Design review of the part built by this model. Coordinates are the model's own, in mm. A direction names the side the tool comes from. Coordinates: 2 decimals unless noted, no trailing zeros. Loops run counter-clockwise (first coordinate to the right, second up) from the corner with the lowest first, then second, coordinate; pieces in that order, holes last. Notation, with made-up numbers: (-25, -29.5) -> (5, -29.5) arc R21 ccw to (5, -22.5) -> close; hole circle Ø4 at (-33.75, 66.5). An arc over 180 degrees is marked (long way). Answer in a Markdown table with one row per item.
```python
from build123d import *

# Parameters (mm, degrees)
BOSS_EXTRUDE1_DEPTH = 12.7
SKETCH2_R           = 3.175
CUT_EXTRUDE1_DEPTH  = 12.7


with BuildPart() as part:
    # Sketch1 → Boss-Extrude1 (new body)
    with BuildSketch(Plane.XY):
        with BuildLine():
            Line((-25.4, 6.391326247), (-25.4, 34.062325918))
            ThreePointArc((-25.4, 34.062325918), (-50.8, 59.462325918), (-76.2, 34.062325918))
            Line((-76.2, 34.062325918), (-101.6, 34.062325918))
            ThreePointArc((-101.6, 34.062325918), (-50.8, 84.862325918), (0, 34.062325918))
            Line((0, 34.062325918), (0, 0))
            Line((0, 0), (0, -43.954875224))
            Line((0, -43.954875224), (-42.435391943, -86.390267166))
            Line((-42.435391943, -86.390267166), (-42.435391943, -180.765389634))
            Line((-42.435391943, -180.765389634), (-67.835391943, -180.765389634))
            Line((-67.835391943, -180.765389634), (-67.835391943, -100.403593512))
            Line((-67.835391943, -100.403593512), (-67.835391943, -75.869242682))
            Line((-67.835391943, -75.869242682), (-25.4, -33.433850739))
            Line((-25.4, -33.433850739), (-25.4, 6.391326247))
        make_face()
    extrude(amount=BOSS_EXTRUDE1_DEPTH)

    # Sketch2 → Cut-Extrude1 (cut)
    with BuildSketch(Plane.XY.offset(12.7)):
        with Locations((-55.135391943, -174.415389634)):
            Circle(SKETCH2_R)
    extrude(amount=-CUT_EXTRUDE1_DEPTH, mode=Mode.SUBTRACT)


solid = part.part
```
(1) Take a section at A-A on z = 10.25. Give the boundary of the cut face in (x, y) (3 decimals).
Evaluation:
| item | result |
|---|---|
| outline | (-101.6, 34.062) -> (-76.2, 34.062) arc R25.4 cw to (-25.4, 34.062) -> (-25.4, -33.434) -> (-67.835, -75.869) -> (-67.835, -180.765) -> (-42.435, -180.765) -> (-42.435, -86.39) -> (0, -43.955) -> (0, 34.062) arc R50.8 ccw to start; hole circle Ø6.35 at (-55.135, -174.415) |
(2) Take a section at D-D on x = -71.5. Give the boundary of the cut face in (y, z).
Evaluation:
| item | result |
|---|---|
| outline | (48.78, 0) -> (80.45, 0) -> (80.45, 12.7) -> (48.78, 12.7) -> close |
(3) Tool access review of faces 4 (the flat face through (-46.915, -54.949, 6.261)), 5 (the cylindrical face through (-50.241, 59.456, 6.261)), 6 (the flat face through (-67.835, -129, 6)): name each direction out of +Z, -Z, +X, -X, +Y, -Y from which nothing blocks a thin tool from reaching the whole face with its end or side.
Evaluation:
| item | result |
|---|---|
| face 4 | +Z, -Z, -X |
| face 5 | +Z, -Z |
| face 6 | +Z, -Z, -X, -Y |
(4) Take a section at C-C on y = -112. Give the boundary of the cut face in (x, z).
Evaluation:
| item | result |
|---|---|
| outline | (-67.84, 0) -> (-42.44, 0) -> (-42.44, 12.7) -> (-67.84, 12.7) -> close |
(5) For pin 1 (10 mm diameter, centred on x = -63.5, y = 56, fed in from -Z); pin 2 (6.5 mm diameter, centred on x = -85.5, z = 9, fed in from -Y); pin 3 (1.5 mm diameter, centred on x = -79.5, z = 9, fed in from +Y); pin 4 (3 mm diameter, centred on x = -90, z = 9.5, fed in from +Y), all flat-tipped, find the tip position at first contact; note any pin that passes through.
Evaluation:
| item | result |
|---|---|
| pin 1 | stops at z = 0 |
| pin 2 | stops at y = 34.06 |
| pin 3 | stops at y = 76.48 |
| pin 4 | stops at y = 68.11 |
(6) Draft analysis for pull direction Y (two halves, no side actions). For faces 1 (the flat face through (0, -4, 6)), 2 (the cylindrical face through (-55.824, -177.515, 6.439)), 3 (the flat face through (-89, 34.062, 6)), state which applies: pulls with the +Y half, pulls with the -Y half, needs draft (parallel to the pull), parting line crosses it, or undercut.
Evaluation:
| item | result |
|---|---|
| face 1 | needs draft |
| face 2 | undercut |
| face 3 | pulls with the -Y half |
(7) To check wall thickness, follow probe 1 along Y at (x, z) = (-54.5, 5); probe 2 along X at (y, z) = (12, 5.75); probe 3 along X at (y, z) = (34.5, 1.75). State the ranges of each line that lie inside material, in increasing order.
Evaluation:
| item | result |
|---|---|
| probe 1 | y = -180.77 to -177.53, -171.3 to -62.53, 59.19 to 84.73 |
| probe 2 | x = -25.4 to 0 |
| probe 3 | x = -101.6 to -76.2, -25.4 to 0 |
(8) Take a section at B-B on x = -47. Give the boundary of the cut face in (y, z), and give its area (3 significant figures).
Evaluation:
| item | result |
|---|---|
| outline | (-180.77, 0) -> (-55.03, 0) -> (-55.03, 12.7) -> (-180.77, 12.7) -> close; (59.18, 0) -> (84.72, 0) -> (84.72, 12.7) -> (59.18, 12.7) -> close |
| area | 1,920 mm² |
